Autodesk Inventor part; units mm, degrees
ref_plane "YZ Plane" through (0, 0, 0) normal (1, 0, 0) x (0, 1, 0)
ref_plane "XZ Plane" through (0, 0, 0) normal (0, 1, 0) x (-1, 0, 0)
ref_plane "XY Plane" through (0, 0, 0) normal (0, 0, 1) x (1, 0, 0)
sketch "Sketch1" plane through (0, 0, 0) normal (0, 0, 1) x (1, 0, 0)
  line L0 (15.5, 0) -> (15.5, 18)
  line L1 (0, 18) -> (0, 0)
  line L2 (7.75, 16.4813) -> (7.75, -1.3789) construction
  arc A0 (5, 11.5) -> (10.5, 11.5) centre (7.75, 11.5) ccw
  line L3 (5, 11.5) -> (5, 18)
  line L4 (10.5, 11.5) -> (10.5, 18)
  line L5 (15.5, 18) -> (10.5, 18)
  line L6 (5, 18) -> (0, 18)
  line L7 (3.5, 0) -> (3.5, 2.8)
  line L8 (5.2, 4.5) -> (10.3, 4.5)
  line L9 (12, 2.8) -> (12, 0)
  line L10 (0, 0) -> (3.5, 0)
  line L11 (12, 0) -> (15.5, 0)
  arc A1 (5.2, 4.5) -> (3.5, 2.8) centre (5.2, 2.8) ccw
  arc A2 (12, 2.8) -> (10.3, 4.5) centre (10.3, 2.8) ccw
  line L12 (1.3235, 11.5) -> (14.2571, 11.5) construction
  point P0 (3.25, 11.5)
  point P1 (12.25, 11.5)
  dimension "d0" = 15.5
  dimension "d1" = 18
  dimension "d3" = 5.5
  dimension "d4" = 6.5
  dimension "d5" = 4.5
  dimension "d6" = 8.5
  dimension "d7" = 1.7
  dimension "d8" = 9
sketch "Sketch2" plane through (0, 0, 0) normal (0, 0, 1) x (1, 0, 0)
  line L0 (0, 18) -> (0, 0)
  line L1 (5, 18) -> (0, 18)
  line L2 (5, 11.5) -> (5, 18)
  arc A0 (5, 11.5) -> (10.5, 11.5) centre (7.75, 11.5) ccw
  line L3 (10.5, 11.5) -> (10.5, 18)
  line L4 (15.5, 18) -> (10.5, 18)
  line L5 (15.5, 0) -> (15.5, 18)
  line L6 (12, 2.8) -> (12, 0)
  line L7 (12, 0) -> (15.5, 0)
  arc A1 (12, 2.8) -> (10.3, 4.5) centre (10.3, 2.8) ccw
  line L8 (5.2, 4.5) -> (10.3, 4.5)
  arc A2 (5.2, 4.5) -> (3.5, 2.8) centre (5.2, 2.8) ccw
  line L9 (3.5, 0) -> (3.5, 2.8)
  line L10 (0, 0) -> (3.5, 0)
extrude "Extrusion1" add sketch "Sketch2" along normal blind 3.5
sketch "Sketch3" plane through (0, 0, 3.5) normal (0, 0, 1) x (1, 0, 0)
  point P0 (0, 0)
  point P1 (3.25, 11.5)
  point P2 (12.25, 11.5)
hole "Hole1" at (3.25, 11.5, 3.5) at (12.25, 11.5, 3.5) direction (0, 0, -1) diameter 1.6 end through all countersink diameter 3 countersink angle 90
sketch "Sketch4" plane through (0, 18, 0) normal (0, 1, 0) x (1, 0, 0)
  line L0 (0, 0) -> (0, -3.5)
  line L1 (0, -1.75) -> (15.5, -1.75) construction
  line L2 (15.5, 0) -> (15.5, -3.5)
  line L3 (5.2, -3.5) -> (10.3, -3.5)
  line L4 (7.75, -3.5) -> (7.75, 0) construction
  point P0 (2.5, -1.75)
  point P1 (13, -1.75)
  dimension "d18" = 10.5
hole "Hole2" at (2.5, 18, 1.75) at (13, 18, 1.75) direction (0, -1, 0) diameter 1.567 depth 4 tip angle 118
sketch "Sketch5" plane through (0, 0, 0) normal (0, -1, 0) x (1, 0, 0)
  line L0 (0, 0) -> (0, 3.5)
  line L1 (0, 1.75) -> (15.5, 1.75) construction
  line L2 (15.5, 0) -> (15.5, 3.5)
  line L3 (5, 3.5) -> (10.5, 3.5)
  line L4 (7.75, 3.5) -> (7.75, 0) construction
  line L5 (10.5, 0) -> (5, 0)
  point P0 (1.75, 1.75)
  point P1 (13.75, 1.75)
  dimension "d26" = 12
hole "Hole3" at (1.75, 0, 1.75) at (13.75, 0, 1.75) direction (0, 1, 0) diameter 1.567 depth 8 tip angle 118
properties part number "mount_motor_side"
Geometry check sheet. Reference: the model listing, model coordinates, mm. A direction names the side the tool comes from. Coordinates: 2 decimals unless noted, no trailing zeros. Order: outer loops, then holes, each group sorted by start corner. A loop starts at its lowest first (then second) coordinate and runs counter-clockwise, first axis right, second up.
Item 1: Scan lines: line 1 along X through (y, z) = (5.75, 1.75); line 2 along X through (y, z) = (15.1, 1.75); line 3 along X through (y, z) = (11.5, 2.1). Record each from-to range of solid material in increasing order.
Item 2: Tool access check on faces 1 (the flat face through (5, 15, 2)), 2 (the cylindrical face through (13.7, 16, 2.1)), 3 (the cylindrical face through (2.445, 4.056, 1.388)), 4 (the flat face through (3.5, 1, 2)). Record the directions out of +Z, -Z, +X, -X, +Y, -Y that give a thin tool (end or side, any length) a straight path to the whole face; none if there is none.
Item 3: Section check C-C (z = 0.6). Enter the section's corners in (x, y).
Item 4: Depth check by flat-ended pin: pin 1 (1.8 mm diameter, centred on x = 13, z = 1.75, fed in from -Y); pin 2 (2 mm diameter, centred on x = 3.25, y = 11.5, fed in from +Z); pin 3 (1.3 mm diameter, centred on x = 2.5, z = 1.75, fed in from +Y); pin 4 (1.3 mm diameter, centred on x = 12.25, y = 11.5, fed in from -Z). Enter the tip coordinate at first touch or a pass-through.
Item 5: Section check A-A (y = 2.25). Enter the section's corners in (x, z), plus the area to 3 significant figures.
Item 6: Section check B-B (y = 15). Enter the section's corners in (x, z), plus the area to 3 significant figures.
Item 7: Mould release check, pull along Y, two halves, no side actions. Record for faces 5 (the cylindrical face through (11.457, 11.604, 1.38)), 6 (the cylindrical face through (3.985, 3.989, 1.726)), 7 (the cylindrical face through (14.445, 4.056, 1.388)), 8 (the conical face through (12.87, 13.61, 1.72)): released by +Y, released by -Y, zero draft, split by the parting line, or undercut.
Item 8: Section check D-D (y = 6.25). Enter the section's corners in (x, z), plus the area to 3 significant figures.
Check sheet entries:
1. line 1: x = 0 to 0.97, 2.53 to 12.97, 14.53 to 15.5
1. line 2: x = 0 to 1.72, 3.28 to 5, 10.5 to 12.22, 13.78 to 15.5
1. line 3: x = 0 to 2.45, 4.05 to 5, 10.5 to 11.45, 13.05 to 15.5
2. face 1: +Z, -Z, +Y
2. face 2: +Y
2. face 3: -Y
2. face 4: +Z, -Z, -Y
3. outline: (0, 0) - (3.5, 0) - (3.5, 2.8) arc R1.7 cw to (5.2, 4.5) - (10.3, 4.5) arc R1.7 cw to (12, 2.8) - (12, 0) - (15.5, 0) - (15.5, 18) - (10.5, 18) - (10.5, 11.5) arc R2.75 cw to (5, 11.5) - (5, 18) - (0, 18) - close; hole circle Ø1.6 at (3.25, 11.5); hole circle Ø1.6 at (12.25, 11.5)
4. pin 1: stops at y = 0
4. pin 2: stops at z = 3
4. pin 3: stops at y = 13.92
4. pin 4: passes through
5. outline: (0, 0) - (3.5, 0) - (3.5, 3.5) - (0, 3.5) - close; (12, 0) - (15.5, 0) - (15.5, 3.5) - (12, 3.5) - close; hole circle Ø1.57 at (1.75, 1.75); hole circle Ø1.57 at (13.75, 1.75)
5. area: 20.6 mm2
6. outline: (0, 0) - (5, 0) - (5, 3.5) - (0, 3.5) - close; (10.5, 0) - (15.5, 0) - (15.5, 3.5) - (10.5, 3.5) - close; hole circle Ø1.57 at (2.5, 1.75); hole circle Ø1.57 at (13, 1.75)
6. area: 31.1 mm2
7. face 5: undercut
7. face 6: released by -Y
7. face 7: zero draft
7. face 8: released by +Y
8. outline: (0, 0) - (15.5, 0) - (15.5, 3.5) - (0, 3.5) - close; hole circle Ø1.57 at (1.75, 1.75); hole circle Ø1.57 at (13.75, 1.75)
8. area: 50.4 mm2
